Autodesk Inventor part; units mm, degrees
ref_plane "YZ Plane" through (0, 0, 0) normal (1, 0, 0) x (0, 1, 0)
ref_plane "XZ Plane" through (0, 0, 0) normal (0, 1, 0) x (-1, 0, 0)
ref_plane "XY Plane" through (0, 0, 0) normal (0, 0, 1) x (1, 0, 0)
sketch "Sketch5" plane through (0, 0, 0) normal (0, 0, 1) x (1, 0, 0)
  line L0 (0, 0) -> (0, 6.35)
  line L1 (0, 6.35) -> (-1.27, 6.35)
  line L2 (-1.27, 6.35) -> (-1.27, 7.9502)
  line L3 (-1.27, 7.9502) -> (29.845, 7.9502)
  line L4 (29.845, 7.9502) -> (29.845, 6.35)
  line L5 (29.845, 6.35) -> (28.575, 6.35)
  line L6 (28.575, 6.35) -> (28.575, 0)
  line L7 (28.575, 0) -> (0, 0)
  line L8 (14.2875, 0) -> (14.2875, 7.9502)
  dimension "d8" = 28.575
  dimension "d9" = 31.115
  dimension "d10" = 6.35
  dimension "d12" = 7.9502
revolve "Revolution2" add sketch "Sketch5" angle 360 about axis through (14.2875, 0, 0) along (0, 1, 0) contours L0 L1 L2 L3 L8 L7
sketch "Sketch6" plane through (14.2875, 7.9502, 0) normal (0, 1, 0) x (1, 0, 0)
  line L0 (-7.3323, 0) -> (-3.6662, 6.35)
  line L1 (-3.6662, 6.35) -> (3.6662, 6.35)
  line L2 (3.6662, 6.35) -> (7.3323, 0)
  line L3 (7.3323, 0) -> (3.6662, -6.35)
  line L4 (3.6662, -6.35) -> (-3.6662, -6.35)
  line L5 (-3.6662, -6.35) -> (-7.3323, 0)
  circle A0 centre (0, 0) radius 15.5575
  circle A1 centre (0, 0) radius 6.8758
  point P0 (-14.2875, 0)
  point P1 (2.637, -6.35)
  point P2 (4.1808, -5.4587)
  point P3 (6.8178, -0.8913)
  point P4 (6.8178, 0.8913)
  point P5 (4.1808, 5.4587)
  point P6 (2.637, 6.35)
  point P7 (-2.637, 6.35)
  point P8 (-4.1808, 5.4587)
  point P9 (-6.8178, 0.8913)
  point P10 (-6.8178, -0.8913)
  point P11 (-4.1808, -5.4587)
  point P12 (-2.637, -6.35)
  dimension "d14" = 12.7
  dimension "d15" = 13.7516
extrude "Extrusion1" cut sketch "Sketch6" against normal through all contours L0 A1 L1 L2 L3 L4 L5
properties part number "part_ Ball Bearing for Thundershaft"
Source: CAD feature listing. Evaluate the final solid. Frame: model axes, mm. A direction names the side the tool comes from. Round coordinates to 2 decimals unless told otherwise and drop trailing zeros. Write each loop counter-clockwise with the first axis right and the second up, starting at its lowest first coordinate (ties: lowest second). Pieces come first, ordered by that corner, then holes. Notation, with made-up numbers: M 36,61.25 L 67,61.25 A12 ccw 67,81.25 Z; hole C 73.25,-12.75 d2. An arc over 180 degrees is marked long. One line per item, written item: value. Start each with the question number.
Item 1: Set-up query: faces 4 (the cylindrical face through (7.41, 4.03, -0.01)), 5 (the flat face through (7, 6.35, -13)), 6 (the flat face through (14, 0, 7)). Return all of +Z, -Z, +X, -X, +Y, -Y with unobstructed straight access to the full face (end or side cutting, diameter ignored); none if empty.
Item 2: Section query A-A (z = 0). Return the cut outline in (x, y) (3 decimals).
Item 3: Section query C-C (x = 14.5). Return the cut outline in (y, z).
Item 4: Mould query, pull axis X, two halves, no side actions, for faces 1 (the flat face through (19.768, 4.031, -3.207)), 2 (the cylindrical face through (28.56, 3.22, 0.63)), 3 (the flat face through (15, 7.95, -7)). Classes: pulls with the +X half, pulls with the -X half, needs draft (parallel to the pull), parting line crosses it, or undercut.
Item 5: Ray query, L1, parallel to Z at x = 14, y = 4.75; L2, parallel to Z at x = 18.5, y = 3.5; L3, parallel to Z at x = 26, y = 4.5. Return the intervals inside material, ascending. Write a range as from..to.
Item 6: Pin query (flat end, axial travel): pin 1 (2 mm diameter, centred on x = 26.5, z = -11, fed in from -Y); pin 2 (1 mm diameter, centred on y = 4.5, z = -6.5, fed in from -X); pin 3 (1.6 mm diameter, centred on x = 14.5, y = 4, fed in from +Z). Return the tip coordinate at first contact, or that it passes through.
Item 7: Section query D-D (z = -12.5). Return the cut outline in (x, y).
Result set:
1. face 4: +Y, -Y
1. face 5: -Y
1. face 6: +Z, -Z, +X, -X, -Y
2. outline: M -1.27,6.35 L 0,6.35 L 0,0 L 7.412,0 L 7.412,7.95 L -1.27,7.95 Z; M 21.163,0 L 28.575,0 L 28.575,6.35 L 29.845,6.35 L 29.845,7.95 L 21.163,7.95 Z
3. outline: M 0,-14.29 L 6.35,-14.29 L 6.35,-15.56 L 7.95,-15.56 L 7.95,-6.35 L 0,-6.35 Z; M 0,6.35 L 7.95,6.35 L 7.95,15.56 L 6.35,15.56 L 6.35,14.29 L 0,14.29 Z
4. face 1: undercut
4. face 2: parting line crosses it
4. face 3: needs draft
5. L1: z = -14.28..-6.35, 6.35..14.28
5. L2: z = -13.65..-5.4, 5.4..13.65
5. L3: z = -8.18..8.18
6. pin 1: stops at y = 6.35
6. pin 2: stops at x = 1.32
6. pin 3: stops at z = 14.29
7. outline: M 5.03,6.35 L 7.37,6.35 L 7.37,0 L 21.21,0 L 21.21,6.35 L 23.55,6.35 L 23.55,7.95 L 5.03,7.95 Z
